Can you work these out from the model? Positions are in its coordinate system, mm. A direction names the side the tool comes from. Coordinates: 2 decimals unless noted, no trailing zeros. Order: outer loops, then holes, each group sorted by start corner. A loop starts at its lowest first (then second) coordinate and runs counter-clockwise, first axis right, second up. Notation, with made-up numbers: (79, 20) -> (103, 20) arc R31 cw to (103, 59) -> close; hole circle Ø7 at (66.25, 12). An arc over 180 degrees is marked (long way). Return JSON: item names as keys, results as strings. Group by question number.
1) Thinking about a two-plate mould opening in Y: for faces 1 (the flat face through (79, 1, 31)), 2 (the flat face through (1, 2, 32)), 3 (the flat face through (48, 9, 2)), which applies, +Y half, -Y half, draft (parallel to the pull), parting line (faces both ways), or undercut?
2) If we section it at A-A, the plane z = 8: Please give me the cut outline in (x, y), then the cut area to 3 significant figures.
3) If we section it at D-D, the plane y = 12.75: Please give me the cut outline in (x, z).
4) If we section it at C-C, the plane x = 62.5: Please give me the cut outline in (y, z), then the cut area to 3 significant figures.
5) If we section it at B-B, the plane z = 32.5: Please give me the cut outline in (x, y).
6) For faces 4 (the flat face through (39, 1, 24)), 5 (the flat face through (49, 18.5, 19)), 6 (the flat face through (95, 9, 20)), which set-ups out of +Z, -Z, +X, -X, +Y, -Y let a thin tool reach every point of the face, with its end or its side?
7) For pin 1 (1.5 mm diameter, centred on y = 6, z = 12.5, fed in from -X); pin 2 (0.6 mm diameter, centred on x = 45, y = 0.5, fed in from +Z); pin 3 (4.5 mm diameter, centred on x = 27, y = 10, fed in from +Z); pin 4 (4 mm diameter, centred on x = 39.5, z = 33.5, fed in from -Y), each with a flat end and sliding along its axis, tell me the tip position at first contact or that it passes through.
8) If I drill on probe 1 along Y at (x, z) = (36.5, 20); probe 2 along X at (y, z) = (12, 21); probe 3 along Y at (x, z) = (31.5, 31), over which ranges is the centre line in solid material (lowest first)? Write a range as from..to.
from build123d import *

# Parameters (mm, degrees)
F0_W     = 97
F0_H     = 18.5
F1_DEPTH = 2
F2_W     = 2
F2_H     = 2
F3_DEPTH = 37
F4_W     = 79
F4_H     = 15
F5_DEPTH = 2


with BuildPart() as f1:
    # F0 (on Top) → F1 (new body)
    with BuildSketch(Plane.XY):
        with Locations((48.5, 9.25)):
            Rectangle(F0_W, F0_H)
    extrude(amount=F1_DEPTH)

    # F2 (on face) → F3 (join)
    with BuildSketch(Plane.XY.offset(2)):
        with Locations((1, 1)):
            Rectangle(F2_W, F2_H)
        Polygon((2, 2), (2, 0), (97, 0), (97, 16.5), (95, 16.5), (95, 2), align=None)
        Polygon((0, 18.5), (0, 2), (2, 2), (2, 16.5), (95, 16.5), (95, 18.5), align=None)
        with Locations((96, 17.5)):
            Rectangle(F2_W, F2_H)
    extrude(amount=F3_DEPTH)

    # F4 (on face) → F5 (cut)
    with BuildSketch(Plane.XZ):
        with Locations((39.5, 31.5)):
            Rectangle(F4_W, F4_H)
    extrude(amount=-F5_DEPTH, mode=Mode.SUBTRACT)


solid = f1.part
Result sheet:
{
 "1": {"face 1": "draft", "face 2": "-Y half", "face 3": "undercut"},
 "2": {"outline": "(0, 0) -> (97, 0) -> (97, 18.5) -> (0, 18.5) -> close; hole (2, 2) -> (95, 2) -> (95, 16.5) -> (2, 16.5) -> close", "area": "446 mm2"},
 "3": {"outline": "(0, 0) -> (97, 0) -> (97, 39) -> (95, 39) -> (95, 2) -> (2, 2) -> (2, 39) -> (0, 39) -> close"},
 "4": {"outline": "(0, 0) -> (18.5, 0) -> (18.5, 39) -> (16.5, 39) -> (16.5, 2) -> (2, 2) -> (2, 24) -> (0, 24) -> close", "area": "155 mm2"},
 "5": {"outline": "(0, 2) -> (2, 2) -> (2, 16.5) -> (95, 16.5) -> (95, 2) -> (79, 2) -> (79, 0) -> (97, 0) -> (97, 18.5) -> (0, 18.5) -> close"},
 "6": {"face 4": "+Z, -X, -Y", "face 5": "+Z, -Z, +X, -X, +Y", "face 6": "+Z"},
 "7": {"pin 1": "stops at x = 0", "pin 2": "stops at z = 24", "pin 3": "stops at z = 2", "pin 4": "stops at y = 16.5"},
 "8": {"probe 1": "y = 0..2, 16.5..18.5", "probe 2": "x = 0..2, 95..97", "probe 3": "y = 16.5..18.5"}
}
